```python
from build123d import *

# Parameters (mm, degrees)
SKETCH_W        = 93
SKETCH_H        = 81
PAD_DEPTH       = 17
SKETCH001_W     = 30.5
SKETCH001_H     = 65.5
POCKET_DEPTH    = 13
SKETCH002_W     = 30.5
SKETCH002_H     = 65
POCKET001_DEPTH = 13
SKETCH003_W     = 13.6458
SKETCH003_H     = 16
POCKET002_DEPTH = 13
SKETCH004_W     = 16.2724
SKETCH004_H     = 17.55
POCKET003_DEPTH = 13
SKETCH005_W     = 15.0186
SKETCH005_H     = 42.9244
POCKET004_DEPTH = 13
SKETCH006_W     = 15
SKETCH006_H     = 25.952942
POCKET005_DEPTH = 12
SKETCH007_W     = 18
SKETCH007_H     = 6.009419
POCKET006_DEPTH = 5
SKETCH009_W     = 7
SKETCH009_H     = 23
POCKET008_DEPTH = 5
SKETCH010_W     = 11.0603
SKETCH010_H     = 11
POCKET009_DEPTH = 1
SKETCH011_W     = 6.5
SKETCH011_H     = 6.5
POCKET010_DEPTH = 17.001
SKETCH014_W     = 16.1
SKETCH014_H     = 12
POCKET011_DEPTH = 5
SKETCH016_R     = 1.6
POCKET012_DEPTH = 12.001
SKETCH017_W     = 90
SKETCH017_H     = 78
SKETCH017_W_2   = 86
SKETCH017_H_2   = 74
PAD001_DEPTH    = 2
SKETCH021_W     = 7.24647
SKETCH021_H     = 11
POCKET013_DEPTH = 3
SKETCH020_R     = 2.8
POCKET014_DEPTH = 2
CHAMFER_SIZE    = 1.5
CHAMFER001_SIZE = 4.5
CHAMFER002_SIZE = 2
FILLET_R        = 1
FILLET001_R     = 5
FILLET002_R     = 5
SKETCH022_W     = 11.3729
SKETCH022_H     = 7.67559
POCKET015_DEPTH = 7
SKETCH023_W     = 9.10313
SKETCH023_H     = 1.48191
POCKET016_DEPTH = 2


with BuildPart() as part:
    # Sketch → Pad (new body)
    with BuildSketch(Plane.XY):
        with Locations((-1.5, 0)):
            Rectangle(SKETCH_W, SKETCH_H)
    extrude(amount=PAD_DEPTH)

    # Sketch001 → Pocket (cut)
    with BuildSketch(Plane.XY.offset(17)):
        with Locations((20.25, 2.25)):
            Rectangle(SKETCH001_W, SKETCH001_H)
    extrude(amount=-POCKET_DEPTH, mode=Mode.SUBTRACT)

    # Sketch002 → Pocket001 (cut)
    with BuildSketch(Plane.XY.offset(17)):
        with Locations((-18.75, 2.5)):
            Rectangle(SKETCH002_W, SKETCH002_H)
    extrude(amount=-POCKET001_DEPTH, mode=Mode.SUBTRACT)

    # Sketch003 → Pocket002 (cut)
    with BuildSketch(Plane.XY.offset(17)):
        with Locations((0, -15)):
            Rectangle(SKETCH003_W, SKETCH003_H)
    extrude(amount=-POCKET002_DEPTH, mode=Mode.SUBTRACT)

    # Sketch004 → Pocket003 (cut)
    with BuildSketch(Plane.XY.offset(17)):
        with Locations((-37.8638, 20.775)):
            Rectangle(SKETCH004_W, SKETCH004_H)
        with Locations((-36.586784, -12.775)):
            Rectangle(SKETCH004_W, SKETCH004_H)
    extrude(amount=-POCKET003_DEPTH, mode=Mode.SUBTRACT)

    # Sketch005 → Pocket004 (cut)
    with BuildSketch(Plane.XY.offset(17)):
        with Locations((0, 12.1505)):
            Rectangle(SKETCH005_W, SKETCH005_H)
    extrude(amount=-POCKET004_DEPTH, mode=Mode.SUBTRACT)

    # Sketch006 → Pocket005 (cut)
    with BuildSketch(Plane(origin=(0, 0, 0), x_dir=(1, 0, 0), z_dir=(0, 0, -1))):
        with Locations((-17.5, 40.976471)):
            Rectangle(SKETCH006_W, SKETCH006_H)
    extrude(amount=-POCKET005_DEPTH, mode=Mode.SUBTRACT)

    # Sketch007 → Pocket006 (cut)
    with BuildSketch(Plane.XY.offset(17)):
        with Locations((-21.9684, -29.726443)):
            Rectangle(SKETCH007_W, SKETCH007_H)
    extrude(amount=-POCKET006_DEPTH, mode=Mode.SUBTRACT)

    # Sketch009 → Pocket008 (cut)
    with BuildSketch(Plane.XY.offset(17)):
        with Locations((38.5, 23.5529)):
            Rectangle(SKETCH009_W, SKETCH009_H)
    extrude(amount=-POCKET008_DEPTH, mode=Mode.SUBTRACT)

    # Sketch010 → Pocket009 (cut)
    with BuildSketch(Plane.XY.offset(17)):
        with Locations((41.12507, 23.7601)):
            Rectangle(SKETCH010_W, SKETCH010_H)
    extrude(amount=-POCKET009_DEPTH, mode=Mode.SUBTRACT)

    # Sketch011 → Pocket010 (cut, through all)
    with BuildSketch(Plane(origin=(0, 0, 0), x_dir=(1, 0, 0), z_dir=(0, 0, -1))):
        with Locations((14.8666, 18.1696)):
            Rectangle(SKETCH011_W, SKETCH011_H)
    extrude(amount=-POCKET010_DEPTH, mode=Mode.SUBTRACT)

    # Sketch014 → Pocket011 (cut)
    with BuildSketch(Plane.YZ.offset(5)):
        with Locations((4.01337, 13)):
            Rectangle(SKETCH014_W, SKETCH014_H)
    extrude(amount=-POCKET011_DEPTH, mode=Mode.SUBTRACT)

    # Sketch016 → Pocket012 (cut, through all)
    with BuildSketch(Plane.XY.offset(12)):
        with Locations((8.75, 30.25)):
            Circle(SKETCH016_R)
        with Locations((31.25, 30.25)):
            Circle(SKETCH016_R)
        with Locations((8.75, -26.25)):
            Circle(SKETCH016_R)
        with Locations((31.25, -26.25)):
            Circle(SKETCH016_R)
    extrude(amount=-POCKET012_DEPTH, mode=Mode.SUBTRACT)

    # Sketch017 → Pad001 (new body)
    with BuildSketch(Plane.XY.offset(17)):
        with Locations((-1.5, 0)):
            Rectangle(SKETCH017_W, SKETCH017_H)
        with Locations((-1.5, 0)):
            Rectangle(SKETCH017_W_2, SKETCH017_H_2, mode=Mode.SUBTRACT)
    extrude(amount=PAD001_DEPTH)

    # Sketch021 → Pocket013 (cut)
    with BuildSketch(Plane.XY.offset(19)):
        with Locations((41.847535, 23.7642)):
            Rectangle(SKETCH021_W, SKETCH021_H)
    extrude(amount=-POCKET013_DEPTH, mode=Mode.SUBTRACT)

    # Sketch020 → Pocket014 (cut)
    with BuildSketch(Plane(origin=(0, 0, 0), x_dir=(1, 0, 0), z_dir=(0, 0, -1))):
        with Locations((8.75, 26.25)):
            Circle(SKETCH020_R)
        with Locations((31.23, 26.25)):
            Circle(SKETCH020_R)
        with Locations((8.75, -30.25)):
            Circle(SKETCH020_R)
        with Locations((31.23, -30.25)):
            Circle(SKETCH020_R)
    extrude(amount=-POCKET014_DEPTH, mode=Mode.SUBTRACT)

    # Chamfer
    chamfer_edges = [part.edges().sort_by_distance(p)[0] for p in [
        (14.8666, -21.4196, 0),
        (18.1166, -18.1696, 0),
        (14.8666, -14.9196, 0),
        (11.6166, -18.1696, 0),
    ]]
    chamfer(chamfer_edges, length=CHAMFER_SIZE)

    # Chamfer001
    chamfer001_edges = [part.edges().sort_by_distance(p)[0] for p in [
        (-17.5, -40.5, 12),
    ]]
    chamfer(chamfer001_edges, length=CHAMFER001_SIZE)

    # Chamfer002
    chamfer002_edges = [part.edges().sort_by_distance(p)[0] for p in [
        (-17.5, -36, 12),
    ]]
    chamfer(chamfer002_edges, length=CHAMFER002_SIZE)

    # Fillet
    fillet_edges = [part.edges().sort_by_distance(p)[0] for p in [
        (41.5, 37, 18),
        (41.5, -37, 18),
        (-44.5, 37, 18),
        (-44.5, -37, 18),
    ]]
    fillet(fillet_edges, radius=FILLET_R)

    # Fillet001
    fillet001_edges = [part.edges().sort_by_distance(p)[0] for p in [
        (-46.5, -39, 18),
        (-46.5, 39, 18),
        (43.5, 39, 18),
        (43.5, -39, 18),
    ]]
    fillet(fillet001_edges, radius=FILLET001_R)

    # Fillet002
    fillet002_edges = [part.edges().sort_by_distance(p)[0] for p in [
        (45, -40.5, 8.5),
        (-48, -40.5, 8.5),
        (-48, 40.5, 8.5),
        (45, 40.5, 8.5),
    ]]
    fillet(fillet002_edges, radius=FILLET002_R)

    # Sketch022 → Pocket015 (cut)
    with BuildSketch(Plane.XY.offset(17)):
        with Locations((0.24661, -25.155595)):
            Rectangle(SKETCH022_W, SKETCH022_H)
    extrude(amount=-POCKET015_DEPTH, mode=Mode.SUBTRACT)

    # Sketch023 → Pocket016 (cut)
    with BuildSketch(Plane.XY.offset(17)):
        with Locations((0.792355, 34.227255)):
            Rectangle(SKETCH023_W, SKETCH023_H)
    extrude(amount=-POCKET016_DEPTH, mode=Mode.SUBTRACT)


solid = part.part
```
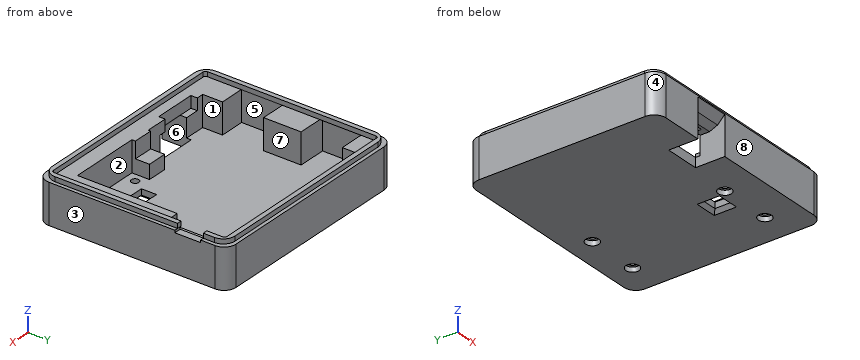
Can you work these out from the model? Positions are in its coordinate system, mm. Face numbers are marked on the shaded views. A direction names the side the tool comes from. Coordinates: 2 decimals unless noted, no trailing zeros. Write each loop counter-clockwise with the first axis right and the second up, starting at its lowest first coordinate (ties: lowest second). Pieces come first, ordered by that corner, then holes. Notation, with made-up numbers: (1.25, -10.75) - (32.25, -10.75) arc R16 cw to (32.25, -1.75) - close; hole circle Ø5 at (-35.5, 2.5). An arc over 180 degrees is marked (long way). Return JSON: item names as keys, results as strings.
Q1. Thinking about a two-plate mould opening in X: for the marked faces 1, 2, 3 and 4, which applies, +X half, -X half, draft (parallel to the pull), parting line (faces both ways), or undercut?
Computed values:
{"face 1": "undercut", "face 2": "undercut", "face 3": "+X half", "face 4": "-X half"}
Q2. Please list where these lines run through material, in increasing order: L1, parallel to Y at x = 31.25, z = 3.4; L2, parallel to X at y = -26.25, z = 1.4; L3, parallel to Y at x = -38.5, z = 7.75. Write a range as from..to.
Computed values:
{"L1": "y = -40.5..-27.85, -24.65..28.65, 31.85..40.5", "L2": "x = -48..5.95, 11.55..28.43, 34.03..45", "L3": "y = -40.5..-21.55, -4..12, 29.55..40.5"}
Q3. If we section it at D-D (x = 23): Please give me the cut outline in (y, z).
Computed values:
{"outline": "(-40.5, 0) - (40.5, 0) - (40.5, 17) - (39, 17) - (39, 19) - (37, 19) - (37, 17) - (35, 17) - (35, 4) - (-30.5, 4) - (-30.5, 17) - (-37, 17) - (-37, 19) - (-39, 19) - (-39, 17) - (-40.5, 17) - close"}
Q4. I'm going to push flat-ended pins straight in: pin 1 Ø4 at (x, y) = (8.75, -26.25) entering from +Z; pin 2 Ø3 at (x, y) = (-19, 1) entering from -Z; pin 3 Ø3.5 at (x, z) = (43, 18) entering from -Y. Where does each tip first touch, or does it pass through?
Computed values:
{"pin 1": "stops at z = 4", "pin 2": "stops at z = 0", "pin 3": "stops at y = -40.25"}
Q5. If we section it at B-B (x = 8.75): Count the separate pieces of the cut face and the enclosed holes in it, then the cut area to 3 significant figures.
Computed values:
{"separate pieces": "3", "enclosed holes": "0", "area": "498 mm2"}
Q6. If we section it at A-A (y = -16): Please give me the cut outline in (x, z).
Computed values:
{"outline": "(-48, 0) - (10.12, 0) - (11.62, 1.5) - (11.62, 4) - (-44.72, 4) - (-44.72, 17) - (-44.5, 17) - (-44.5, 19) - (-46.5, 19) - (-46.5, 17) - (-48, 17) - close; (18.12, 1.5) - (19.62, 0) - (45, 0) - (45, 17) - (43.5, 17) - (43.5, 19) - (41.5, 19) - (41.5, 17) - (35.5, 17) - (35.5, 4) - (18.12, 4) - close"}
Q7. On a 3-axis mill with a long thin cutter (end or side, diameter ignored), from which of +Z, -Z, +X, -X, +Y, -Y can I reach the whole of each face in a straight line? I mean the marked faces 5, 6, 7 and 8. Say none if no direction works.
Computed values:
{"face 5": "none", "face 6": "-Z, -Y", "face 7": "+Z", "face 8": "+Z, -Z, +X, -X, -Y"}
